```python
from build123d import *

# Parameters (mm, degrees)
SKETCH_1_W          = 255
SKETCH_1_H          = 138
EXTRUDE_1_DEPTH     = 1
CUT_EXTRUDE_1_DEPTH = 188.88626879
SKETCH_5_W          = 3
SKETCH_5_H          = 20
EXTRUDE_3_DEPTH     = 1
SKETCH_6_R          = 1
CUT_EXTRUDE_3_DEPTH = 190.934857254
CUT_EXTRUDE_5_DEPTH = 190.934857254
FILLET_1_R          = 1


with BuildPart() as part:
    # 草图1 → 凸台-拉伸1 (new body)
    with BuildSketch(Plane(origin=(0, 0, 0), x_dir=(1, 0, 0), z_dir=(0, 1, 0))):
        with Locations((0, -69)):
            Rectangle(SKETCH_1_W, SKETCH_1_H)
    extrude(amount=EXTRUDE_1_DEPTH)

    # 草图2 → 切除-拉伸1 (cut, through all)
    with BuildSketch(Plane(origin=(0, 1, 0), x_dir=(1, 0, 0), z_dir=(0, 1, 0))):
        with BuildLine():
            Line((-115.5, 0), (115.5, 0))
            ThreePointArc((115.5, 0), (0, -67.533957913), (-115.5, 0))
        make_face()
    extrude(amount=-CUT_EXTRUDE_1_DEPTH, mode=Mode.SUBTRACT)

    # 草图5 → 凸台-拉伸3 (add)
    with BuildSketch(Plane(origin=(0, 1, 0), x_dir=(1, 0, 0), z_dir=(0, 1, 0))):
        with Locations((-129, -25)):
            Rectangle(SKETCH_5_W, SKETCH_5_H)
        with Locations((-129, -70)):
            Rectangle(SKETCH_5_W, SKETCH_5_H)
        with Locations((129, -25)):
            Rectangle(SKETCH_5_W, SKETCH_5_H)
        with Locations((-129, -115)):
            Rectangle(SKETCH_5_W, SKETCH_5_H)
        with Locations((129, -115)):
            Rectangle(SKETCH_5_W, SKETCH_5_H)
        with Locations((129, -70)):
            Rectangle(SKETCH_5_W, SKETCH_5_H)
    extrude(amount=-EXTRUDE_3_DEPTH)

    # 草图6 → 切除-拉伸3 (cut, through all)
    with BuildSketch(Plane(origin=(0, 1, 0), x_dir=(1, 0, 0), z_dir=(0, 1, 0))):
        with Locations((-127.5, -14)):
            Circle(SKETCH_6_R)
        with Locations((-127.5, -36)):
            Circle(SKETCH_6_R)
        with Locations((127.5, -36)):
            Circle(SKETCH_6_R)
        with Locations((127.5, -14)):
            Circle(SKETCH_6_R)
        with Locations((-127.5, -59)):
            Circle(SKETCH_6_R)
        with Locations((-127.5, -81)):
            Circle(SKETCH_6_R)
        with Locations((-127.5, -104)):
            Circle(SKETCH_6_R)
        with Locations((-127.5, -126)):
            Circle(SKETCH_6_R)
        with Locations((127.5, -126)):
            Circle(SKETCH_6_R)
        with Locations((127.5, -104)):
            Circle(SKETCH_6_R)
        with Locations((127.5, -81)):
            Circle(SKETCH_6_R)
        with Locations((127.5, -59)):
            Circle(SKETCH_6_R)
    extrude(amount=-CUT_EXTRUDE_3_DEPTH, mode=Mode.SUBTRACT)

    # 草图7 → 切除-拉伸5 (cut, through all)
    with BuildSketch(Plane(origin=(0, 1, 0), x_dir=(1, 0, 0), z_dir=(0, 1, 0))):
        with BuildLine():
            Line((-96, -44.259051802), (-96, -119))
            ThreePointArc((-96, -119), (-105, -128), (-114, -119))
            Line((-114, -119), (-114, -44.259051802))
            ThreePointArc((-114, -44.259051802), (-105, -35.259051802), (-96, -44.259051802))
        make_face()
        with BuildLine():
            Line((-66, -66.672094237), (-66, -119))
            ThreePointArc((-66, -119), (-75, -128), (-84, -119))
            Line((-84, -119), (-84, -66.672094237))
            ThreePointArc((-84, -66.672094237), (-75, -57.672094237), (-66, -66.672094237))
        make_face()
        with BuildLine():
            Line((-36, -79.698100888), (-36, -119))
            ThreePointArc((-36, -119), (-45, -128), (-54, -119))
            Line((-54, -119), (-54, -79.698100888))
            ThreePointArc((-54, -79.698100888), (-45, -70.698100888), (-36, -79.698100888))
        make_face()
        with BuildLine():
            Line((-6, -85.789722464), (-6, -119))
            ThreePointArc((-6, -119), (-15, -128), (-24, -119))
            Line((-24, -119), (-24, -85.789722464))
            ThreePointArc((-24, -85.789722464), (-15, -76.789722464), (-6, -85.789722464))
        make_face()
        with BuildLine():
            Line((6, -85.789722464), (6, -119))
            ThreePointArc((6, -119), (15, -128), (24, -119))
            Line((24, -119), (24, -85.789722464))
            ThreePointArc((24, -85.789722464), (15, -76.789722464), (6, -85.789722464))
        make_face()
        with BuildLine():
            Line((36, -79.698100888), (36, -119))
            ThreePointArc((36, -119), (45, -128), (54, -119))
            Line((54, -119), (54, -79.698100888))
            ThreePointArc((54, -79.698100888), (45, -70.698100888), (36, -79.698100888))
        make_face()
        with BuildLine():
            Line((66, -66.672094237), (66, -119))
            ThreePointArc((66, -119), (75, -128), (84, -119))
            Line((84, -119), (84, -66.672094237))
            ThreePointArc((84, -66.672094237), (75, -57.672094237), (66, -66.672094237))
        make_face()
        with BuildLine():
            Line((96, -44.259051802), (96, -119))
            ThreePointArc((96, -119), (105, -128), (114, -119))
            Line((114, -119), (114, -44.259051802))
            ThreePointArc((114, -44.259051802), (105, -35.259051802), (96, -44.259051802))
        make_face()
    extrude(amount=-CUT_EXTRUDE_5_DEPTH, mode=Mode.SUBTRACT)

    # 圆角1
    fillet_1_edges = [part.edges().sort_by_distance(p)[0] for p in [
        (-127.5, 0.5, 58),
        (115.5, 0.5, 0),
        (-115.5, 0.5, 0),
        (-130.5, 0.5, 35),
        (-130.5, 0.5, 15),
        (130.5, 0.5, 15),
        (130.5, 0.5, 35),
        (-130.5, 0.5, 80),
        (-130.5, 0.5, 60),
        (-130.5, 0.5, 125),
        (-130.5, 0.5, 105),
        (130.5, 0.5, 105),
        (130.5, 0.5, 125),
        (-127.5, 0.5, 0),
        (127.5, 0.5, 0),
        (127.5, 0.5, 138),
        (-127.5, 0.5, 138),
        (130.5, 0.5, 60),
        (130.5, 0.5, 80),
    ]]
    fillet(fillet_1_edges, radius=FILLET_1_R)


solid = part.part
```
Part model, mm, in its own coordinate system. A direction names the side the tool comes from. Coordinates: 2 decimals unless noted, no trailing zeros. Write each loop counter-clockwise with the first axis right and the second up, starting at its lowest first coordinate (ties: lowest second). Pieces come first, ordered by that corner, then holes.
Item 1: Probe line 1 (X direction, y = 0.45, z = 38.5); line 2 (X direction, y = 0.1, z = 69); line 3 (X direction, y = 0.25, z = 55). List the from-to ranges inside material, lowest first.
Item 2: Slice it at D-D (z = 28.5). Write the cut outline in (x, y).
Item 3: Pin check, flat tips, straight feed: pin 1 (0.5 mm diameter, centred on y = 0.5, z = 104, fed in from +X); pin 2 (3 mm diameter, centred on x = 34, z = 91.5, fed in from -Y). Stop position of each tip, or through.
Item 4: Slice it at A-A (z = 50.5). Write the cut outline in (x, y).
Item 5: Which spindle directions (+Z, -Z, +X, -X, +Y, -Y) get a long thin tool onto all of the face, cutting with end or side? Do faces 4 (the face through (-2, 0, 83)), 5 (the face through (-44.802, 0.507, 127.998)). Say none if no direction does.
Item 6: Mould opens along Z. For faces 1 (the face through (44.802, 0.507, 127.998)), 2 (the face through (-2, 1, 83)), 3 (the face through (1.96, 0.51, 67.52)) say: released by +Z, released by -Z, zero draft, split by the parting line, or undercut.
Item 7: Slice it at C-C (y = 0.5). Count the separate pieces of the cut face and the enclosed holes in it, and give its area (3 significant figures).
Item 8: Slice it at B-B (x = -106). Write the cut outline in (y, z), and give its area (3 significant figures).
Results found:
1. line 1: x = -127.5 to -111.92, -98.08 to -82.78, 82.78 to 98.08, 111.92 to 127.5
1. line 2: x = -130.5 to -114, -96 to -84, -66 to 66, 84 to 96, 114 to 130.5
1. line 3: x = -127.5 to -114, -96 to -56.26, 56.26 to 96, 114 to 127.5
2. outline: (-130.5, 0) - (-93.93, 0) - (-93.93, 1) - (-130.5, 1) - close; (93.93, 0) - (130.5, 0) - (130.5, 1) - (93.93, 1) - close
3. pin 1: stops at x = 126.53
3. pin 2: stops at y = 0
4. outline: (-127.5, 0) - (-114, 0) - (-114, 1) - (-127.5, 1) - close; (-96, 0) - (-65, 0) - (-65, 1) - (-96, 1) - close; (65, 0) - (96, 0) - (96, 1) - (65, 1) - close; (114, 0) - (127.5, 0) - (127.5, 1) - (114, 1) - close
5. face 4: +Z, -Z, +X, -X, -Y
5. face 5: +Y, -Y
6. face 1: undercut
6. face 2: zero draft
6. face 3: released by -Z
7. separate pieces: 1
7. enclosed holes: 8
7. area: 15,200 mm2
8. outline: (0, 14.56) - (1, 14.56) - (1, 35.31) - (0, 35.31) - close; (0, 127.94) - (1, 127.94) - (1, 138) - (0, 138) - close
8. area: 30.8 mm2
